Geometry check sheet. Reference: the model listing, model coordinates, mm. A direction names the side the tool comes from. Round coordinates to 2 decimals unless told otherwise and drop trailing zeros. Write each loop counter-clockwise with the first axis right and the second up, starting at its lowest first coordinate (ties: lowest second). Pieces come first, ordered by that corner, then holes. Notation, with made-up numbers: (9.5, 34) - (45.5, 34) arc R28 ccw to (45.5, 66) - close; hole circle Ø8 at (-35.5, 8.5). An arc over 180 degrees is marked (long way). Return JSON: item names as keys, results as strings.
```python
from build123d import *

# Parameters (mm, degrees)
SKETCH1_R           = 1.25
SKETCH1_R_2         = 1.15
BOSS_EXTRUDE1_DEPTH = 3
FILLET2_R           = 1


with BuildPart() as part:
    # Sketch1 → Boss-Extrude1 (new body)
    with BuildSketch(Plane.XY):
        Polygon((-27.25, 21), (-27.25, 0), (-27.25, -15), (-9.25, -15), (-9.25, 3), (-14.25, 3), (-14.25, 21), align=None)
        with Locations((-21, 17.5)):
            Circle(SKETCH1_R, mode=Mode.SUBTRACT)
        with Locations((-21, 10.5)):
            Circle(SKETCH1_R, mode=Mode.SUBTRACT)
        with Locations((-21, 3.5)):
            Circle(SKETCH1_R, mode=Mode.SUBTRACT)
        with Locations((-13.5, -10.3)):
            Circle(SKETCH1_R_2, mode=Mode.SUBTRACT)
        with Locations((-24.5, -10.3)):
            Circle(SKETCH1_R_2, mode=Mode.SUBTRACT)
    extrude(amount=BOSS_EXTRUDE1_DEPTH)

    # Fillet2
    fillet2_edges = [part.edges().sort_by_distance(p)[0] for p in [
        (-20.75, 21, 0),
        (-14.25, 12, 3),
        (-20.75, 21, 3),
        (-14.25, 12, 0),
        (-11.75, 3, 0),
        (-9.25, -6, 0),
        (-18.25, -15, 0),
        (-27.25, 3, 3),
        (-27.25, 3, 0),
    ]]
    fillet(fillet2_edges, radius=FILLET2_R)


solid = part.part
```
(1) Section check D-D, the plane x = -24.5. Enter the section's corners in (y, z), plus the area to 3 significant figures.
Response values:
{"outline": "(-15, 1) arc R1 ccw to (-14, 0) - (-11.45, 0) - (-11.45, 3) - (-15, 3) - close; (-9.15, 0) - (20, 0) arc R1 ccw to (21, 1) - (21, 2) arc R1 ccw to (20, 3) - (-9.15, 3) - close", "area": "100 mm^2"}
(2) Release check for a two-part mould opening along X. For faces 1 (the face through (-9.25, -6, 2)), 2 (the face through (-18, -15, 2)), 3 (the face through (-19.845, 3.021, 1.479)) record: pulls with the +X half, pulls with the -X half, needs draft (parallel to the pull), parting line crosses it, or undercut.
Response values:
{"face 1": "pulls with the +X half", "face 2": "needs draft", "face 3": "undercut"}
(3) Access from +Z, -Z, +X, -X, +Y, -Y to the whole of each face (thin tool, end or side, straight path). Record for faces 4 (the face through (-23.97, -11.32, 1.48)), 5 (the face through (-14.535, 12.126, 2.699)), 6 (the face through (-9.535, -5.874, 0.301)), 7 (the face through (-14.25, 11.9, 1.5)), 8 (the face through (-14.535, 11.633, 0.301)).
Response values:
{"face 4": "+Z, -Z", "face 5": "+Z, +X, +Y", "face 6": "-Z, +X, +Y, -Y", "face 7": "+Z, -Z, +X, +Y", "face 8": "-Z, +X, +Y"}
(4) Section check B-B, the plane x = -21. Enter the section's corners in (y, z), plus the area to 3 significant figures.
Response values:
{"outline": "(-15, 1) arc R1 ccw to (-14, 0) - (2.25, 0) - (2.25, 3) - (-15, 3) - close; (4.75, 0) - (9.25, 0) - (9.25, 3) - (4.75, 3) - close; (11.75, 0) - (16.25, 0) - (16.25, 3) - (11.75, 3) - close; (18.75, 0) - (20, 0) arc R1 ccw to (21, 1) - (21, 2) arc R1 ccw to (20, 3) - (18.75, 3) - close", "area": "84.9 mm^2"}
(5) Material ranges on line 1 along Y through (x, z) = (-21, 0.95); line 2 along Y through (x, z) = (-24.5, 1.9); line 3 along Y through (x, z) = (-21, 2.55), recorded low to high. Write a range as [from, to].
Response values:
{"line 1": "y = [-15, 2.25], [4.75, 9.25], [11.75, 16.25], [18.75, 21]", "line 2": "y = [-15, -11.45], [-9.15, 21]", "line 3": "y = [-15, 2.25], [4.75, 9.25], [11.75, 16.25], [18.75, 20.84]"}
(6) Section check A-A, the plane y = -10.3. Enter the section's corners in (x, z).
Response values:
{"outline": "(-27.25, 1) arc R1 ccw to (-26.25, 0) - (-25.65, 0) - (-25.65, 3) - (-26.25, 3) arc R1 ccw to (-27.25, 2) - close; (-23.35, 0) - (-14.65, 0) - (-14.65, 3) - (-23.35, 3) - close; (-12.35, 0) - (-10.25, 0) arc R1 ccw to (-9.25, 1) - (-9.25, 3) - (-12.35, 3) - close"}
(7) Gauge pin test, flat ends, axial feed: pin 1 (0.6 mm diameter, centred on x = -11, z = 1.5, fed in from +Y); pin 2 (0.8 mm diameter, centred on y = 13, z = 1.5, fed in from +X). Record the tip position at first contact, or that the pin passes through.
Response values:
{"pin 1": "stops at y = 3", "pin 2": "stops at x = -14.25"}
(8) Section check C-C, the plane z = 1.35. Enter the section's corners in (x, y).
Response values:
{"outline": "(-27.25, -15) - (-9.25, -15) - (-9.25, 3) - (-14.25, 3) - (-14.25, 21) - (-27.25, 21) - close; hole circle Ø2.3 at (-24.5, -10.3); hole circle Ø2.5 at (-21, 3.5); hole circle Ø2.5 at (-21, 10.5); hole circle Ø2.5 at (-21, 17.5); hole circle Ø2.3 at (-13.5, -10.3)"}
